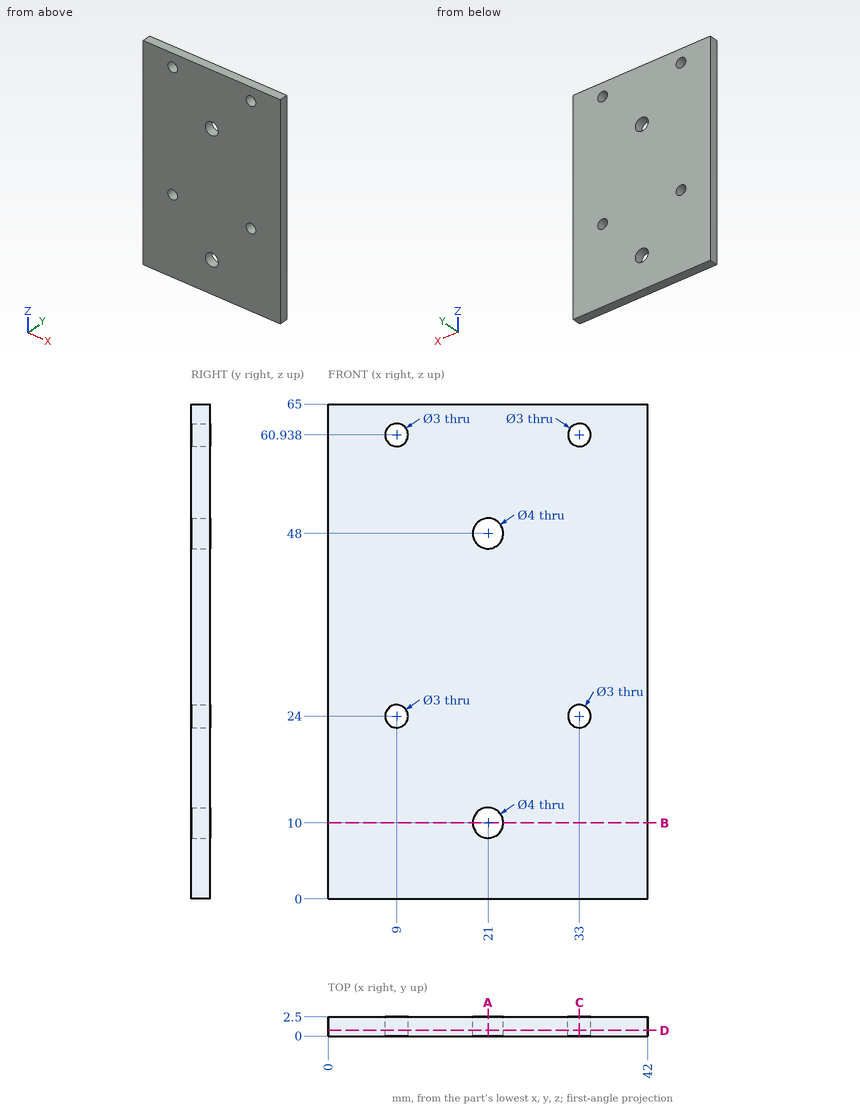
Here's the drawing with two shaded views (mm, measured from the low corner). I have some questions. Coordinates: 2 decimals unless noted, no trailing zeros. Loops run counter-clockwise (first coordinate to the right, second up) from the corner with the lowest first, then second, coordinate; pieces in that order, holes last. Notation, with made-up numbers: M 73,27.5 L 113,27.5 A20 ccw 113,51.5 Z; hole C 19,-14 d6. An arc over 180 degrees is marked long. Return JSON: item names as keys, results as strings. Group by question number.
Item 1: Imagine slicing it at B-B (z = 10). Please give me the cut outline in (x, y).
Item 2: If I drill on L1, parallel to Z at x = 33, y = 1.1; L2, parallel to Z at x = 21, y = 0.65, over which ranges is the centre line in solid material (lowest first)? Write a range as from..to.
Item 3: Imagine slicing it at C-C (x = 33). Please give me the cut outline in (y, z).
Item 4: Imagine slicing it at A-A (x = 21). Please give me the cut outline in (y, z).
Item 5: Imagine slicing it at D-D (y = 0.75). Please give me the cut outline in (x, z), and give its area (3 significant figures).
Verdict:
{
 "1": {"outline": "M 0,0 L 19,0 L 19,2.5 L 0,2.5 Z; M 23,0 L 42,0 L 42,2.5 L 23,2.5 Z"},
 "2": {"L1": "z = 0..22.5, 25.5..59.44, 62.44..65", "L2": "z = 0..8, 12..46, 50..65"},
 "3": {"outline": "M 0,0 L 2.5,0 L 2.5,22.5 L 0,22.5 Z; M 0,25.5 L 2.5,25.5 L 2.5,59.44 L 0,59.44 Z; M 0,62.44 L 2.5,62.44 L 2.5,65 L 0,65 Z"},
 "4": {"outline": "M 0,0 L 2.5,0 L 2.5,8 L 0,8 Z; M 0,12 L 2.5,12 L 2.5,46 L 0,46 Z; M 0,50 L 2.5,50 L 2.5,65 L 0,65 Z"},
 "5": {"outline": "M 0,0 L 42,0 L 42,65 L 0,65 Z; hole C 9,24 d3; hole C 9,60.94 d3; hole C 21,10 d4; hole C 21,48 d4; hole C 33,24 d3; hole C 33,60.94 d3", "area": "2,680 mm^2"}
}
